Autodesk Inventor part; units mm, degrees
ref_plane "YZ Plane" through (0, 0, 0) normal (1, 0, 0) x (0, 1, 0)
ref_plane "XZ Plane" through (0, 0, 0) normal (0, 1, 0) x (-1, 0, 0)
ref_plane "XY Plane" through (0, 0, 0) normal (0, 0, 1) x (1, 0, 0)
sketch "Sketch1" plane through (0, 0, 0) normal (0, 0, 1) x (1, 0, 0)
  line L0 (35.56, 293.2939) -> (25.4, 0)
  line L1 (35.56, 293.2939) -> (-650.24, 293.2939)
  line L2 (-650.24, 293.2939) -> (-270.7381, 0)
  arc A0 (19.0462, 0) -> (-260.3538, 0) centre (-120.6538, 0) ccw
  line L3 (-270.7381, 0) -> (-260.3538, 0)
  line L4 (19.0462, 0) -> (25.4, 0)
  point P0 (0, 0)
  dimension "d2" = 293.2939
  dimension "d3" = 35.56
  dimension "d4" = 25.4
  dimension "d5" = 685.8
  dimension "d8" = 279.4
  dimension "d11" = 6.35
  dimension "d12" = 6.35
extrude "Extrusion1" add sketch "Sketch1" along normal blind 6.35
sketch "Sketch2" plane through (0, 0, 6.35) normal (0, 0, 1) x (1, 0, 0)
  line L0 (25.4, 0) -> (35.56, 293.2939)
  line L1 (28.3345, 268.129) -> (34.6806, 267.9092)
  line L2 (27.8948, 255.4366) -> (34.241, 255.2168)
  line L3 (23.498, 128.5127) -> (29.8442, 128.2929)
  line L4 (23.0583, 115.8204) -> (29.4045, 115.6005)
  line L5 (23.0583, 115.8204) -> (23.498, 128.5127)
  line L6 (27.8948, 255.4366) -> (28.3345, 268.129)
  point P0 (0, 0)
  dimension "d21" = 12.7
  dimension "d23" = 12.7
  dimension "d24" = 25.4
  dimension "d25" = 127
extrude "Extrusion2" cut sketch "Sketch2" against normal blind 6.35
sketch "Sketch3" plane through (0, 0, 6.35) normal (0, 0, 1) x (1, 0, 0)
  line L0 (-650.24, 293.2939) -> (-270.7381, 0)
  line L1 (-589.9473, 246.6974) -> (-586.0643, 251.7218)
  line L2 (-576.0155, 243.9557) -> (-579.8986, 238.9313)
  line L3 (-334.8449, 57.5696) -> (-338.7279, 52.5452)
  line L4 (-324.7961, 49.8035) -> (-328.6792, 44.7792)
  line L5 (-586.0643, 251.7218) -> (-576.0155, 243.9557)
  line L6 (-334.8449, 57.5696) -> (-324.7961, 49.8035)
  point P0 (0, 0)
  dimension "d28" = 6.35
  dimension "d29" = 12.7
  dimension "d30" = 12.7
  dimension "d31" = 76.2
  dimension "d32" = 304.8
extrude "Extrusion3" cut sketch "Sketch3" against normal blind 6.35
properties part number "Funneling2" material "Polycarbonate, Clear"
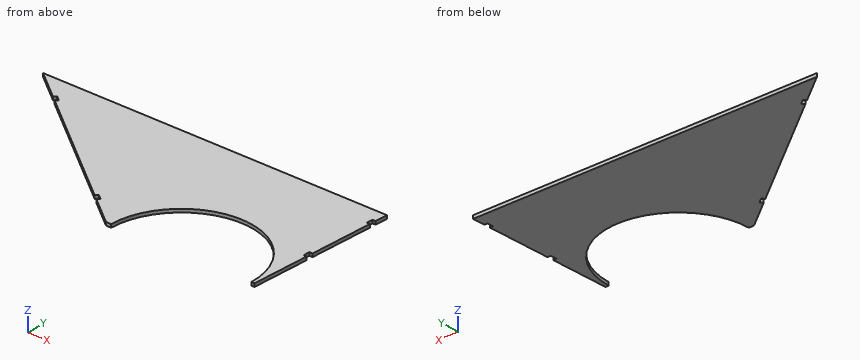
Can you work these out from the model? Positions are in its coordinate system, mm. Round coordinates to 2 decimals unless told otherwise and drop trailing zeros. Loops run counter-clockwise (first coordinate to the right, second up) from the corner with the lowest first, then second, coordinate; pieces in that order, holes last.
Item 1: Will this pin go through, and if not, where does the flat tip stop? pin 1 Ø2 at (y, z) = (125.5, 3.5) entering from +X.
Item 2: Suppose I cut it at B-B, the plane y = 105. Write out the boundary of the cut face in (x, z), then the cut area to 3 significant figures.
Item 3: Suppose I cut it at D-D, the plane x = -299. Write out the boundary of the cut face in (y, z), then the cut area to 3 significant figures.
Item 4: Suppose I cut it at A-A, the plane y = 36.5. Write out the boundary of the cut face in (x, z).
Item 5: Suppose I cut it at C-C, the plane z = 3. Write out the boundary of the cut face in (x, y).
Item 6: Please list where these lines run through material, in increasing order: L1, parallel to X at y = 129, z = 0.5; L2, parallel to X at y = 47, z = 4; L3, parallel to Y at x = -201, z = 2.5.
Reported:
1. pin 1: stops at x = 23.43
2. outline: (-406.6, 0) - (-212.8, 0) - (-212.8, 6.35) - (-406.6, 6.35) - close; (-28.51, 0) - (29.04, 0) - (29.04, 6.35) - (-28.51, 6.35) - close
2. area: 1,600 mm2
3. outline: (21.84, 0) - (293.29, 0) - (293.29, 6.35) - (21.84, 6.35) - close
3. area: 1,720 mm2
4. outline: (-317.97, 0) - (-255.5, 0) - (-255.5, 6.35) - (-317.97, 6.35) - close; (14.19, 0) - (26.66, 0) - (26.66, 6.35) - (14.19, 6.35) - close
5. outline: (-650.24, 293.29) - (-589.95, 246.7) - (-586.06, 251.72) - (-576.02, 243.96) - (-579.9, 238.93) - (-338.73, 52.55) - (-334.84, 57.57) - (-324.8, 49.8) - (-328.68, 44.78) - (-270.74, 0) - (-260.35, 0) arc R139.7 cw to (19.05, 0) - (25.4, 0) - (29.4, 115.6) - (23.06, 115.82) - (23.5, 128.51) - (29.84, 128.29) - (34.24, 255.22) - (27.89, 255.44) - (28.33, 268.13) - (34.68, 267.91) - (35.56, 293.29) - close
6. L1: x = -437.66 to -174.27, -67.03 to 29.87
6. L2: x = -326.96 to -252.21, 10.9 to 27.03
6. L3: y = 114.28 to 293.29
